from build123d import *

# Parameters (mm, degrees)
SKETCH1_W           = 30
SKETCH1_H           = 11.167486893
SKETCH1_R           = 27.5
SKETCH1_R_2         = 3.25
SKETCH1_R_3         = 12
BOSS_EXTRUDE1_DEPTH = 25.4
SKETCH2_R           = 2.45745
CUT_EXTRUDE1_DEPTH  = 31


with BuildPart() as part:
    # Sketch1 → Boss-Extrude1 (new body)
    # profile 1 of 4: a face of its own
    with BuildSketch(Plane.XY):
        with Locations((-100, -5.583743447)):
            Rectangle(SKETCH1_W, SKETCH1_H)
    # profile 2 of 4: a face of its own
    with BuildSketch(Plane.XY):
        with BuildLine():
            Line((-85, -11.167486893), (-85, -37.625000004))
            ThreePointArc((-85, -37.625000004), (-57.5, -10.125000004), (-30, -37.625000004))
            Line((-30, -37.625000004), (-30, -11.167486893))
            Line((-30, -11.167486893), (-30, 0))
            Line((-30, 0), (-85, 0))
            Line((-85, 0), (-85, -11.167486893))
        make_face()
    # profile 3 of 4: a face of its own
    with BuildSketch(Plane.XY):
        with Locations((-57.5, -37.625000004)):
            Circle(SKETCH1_R)
        with Locations((-58.583096057, -15.151083947)):
            Circle(SKETCH1_R_2, mode=Mode.SUBTRACT)
        with Locations((-38.578565801, -25.450053276)):
            Circle(SKETCH1_R_2, mode=Mode.SUBTRACT)
        with Locations((-37.495469744, -47.923969333)):
            Circle(SKETCH1_R_2, mode=Mode.SUBTRACT)
        with Locations((-56.416903943, -60.098916061)):
            Circle(SKETCH1_R_2, mode=Mode.SUBTRACT)
        with Locations((-76.421434199, -49.799946732)):
            Circle(SKETCH1_R_2, mode=Mode.SUBTRACT)
        with Locations((-77.504530256, -27.326030675)):
            Circle(SKETCH1_R_2, mode=Mode.SUBTRACT)
        with Locations((-57.5, -37.625000004)):
            Circle(SKETCH1_R_3, mode=Mode.SUBTRACT)
    # profile 4 of 4: a face of its own
    with BuildSketch(Plane.XY):
        with Locations((-15, -5.583743447)):
            Rectangle(SKETCH1_W, SKETCH1_H)
    extrude(amount=BOSS_EXTRUDE1_DEPTH)

    # Sketch2 → Cut-Extrude1 (cut)
    with BuildSketch(Plane(origin=(0, 0, 0), x_dir=(1, 0, 0), z_dir=(0, 1, 0))):
        with Locations(Location((-93.73, -12.7, 0), (0, 0, 270))):
            Circle(SKETCH2_R)
        with Locations(Location((-106.43, -12.7, 0), (0, 0, 270))):
            Circle(SKETCH2_R)
        with Locations(Location((-17.53, -12.7, 0), (0, 0, 270))):
            Circle(SKETCH2_R)
        with Locations(Location((-4.83, -12.7, 0), (0, 0, 270))):
            Circle(SKETCH2_R)
    extrude(amount=-CUT_EXTRUDE1_DEPTH, mode=Mode.SUBTRACT)


solid = part.part
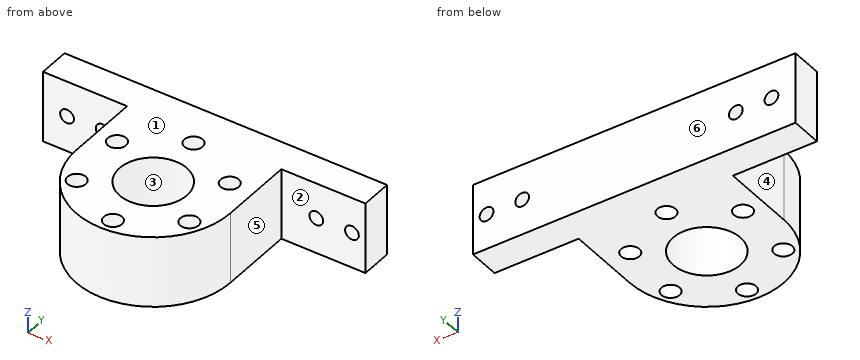
CAD build for the part. Positions are in the model's coordinates, mm. Face numbers are marked on the shaded views. A direction names the side the tool comes from. Round coordinates to 2 decimals unless told otherwise and drop trailing zeros. Write each loop counter-clockwise with the first axis right and the second up, starting at its lowest first coordinate (ties: lowest second). Pieces come first, ordered by that corner, then holes. Notation, with made-up numbers: M 65.5,-27 L 123.5,-27 A23 cw 123.5,-8 Z; hole C 2.5,-2 d9. An arc over 180 degrees is marked long. Use a Markdown table: item, result. Add a question column.
1. Slice it at A-A on x = -106.43. Give the cut face in (y, z).
2. Flat gauge pins, fed straight in: P1, Ø12, axis at x = -35.5, z = 11.5, coming from the -Y side; P2, Ø2, axis at y = -28, z = 13.5, coming from the -X side; P3, Ø12, axis at x = -93, y = -46.5, coming from the -Z side; P4, Ø6.5, axis at x = -17.53, z = 12.7, coming from the -Y side. Where does each tip first touch, or does it go through?
3. Pull direction Y, two halves, no side cores. Call the marked faces 1, 2 and 3: released by +Y, released by -Y, zero draft, split by the parting line, or undercut.
4. Drill centre lines: probe 1 along X at (y, z) = (-4, 12.7); probe 2 along Y at (x, z) = (-57.5, 12.5) (3 decimals); probe 3 along Y at (x, z) = (-55, 21.25). Where is each one in solid material? Low to high.
5. 3-axis set-ups, long thin cutter, end or side, ignore diameter. For the marked faces 4, 5 and 6: which of +Z, -Z, +X, -X, +Y, -Y reach the whole face in a straight line?
6. Slice it at C-C on x = -78. Give the cut face in (y, z), then the cut area to 3 significant figures.
7. Slice it at D-D on y = -35.5. Give the cut face in (x, z), then the cut area to 3 significant figures.
8. Slice it at B-B on y = -4.5. Give the cut face in (x, z), then the cut area to 3 significant figures.
Reply:
| question | item | result |
|---|---|---|
| 1 | outline | M -11.17,0 L 0,0 L 0,10.24 L -11.17,10.24 Z; M -11.17,15.16 L 0,15.16 L 0,25.4 L -11.17,25.4 Z |
| 2 | P1 | stops at y = -59.99 |
| 2 | P2 | stops at x = -85 |
| 2 | P3 | passes through |
| 2 | P4 | stops at y = -11.17 |
| 3 | face 1 | zero draft |
| 3 | face 2 | released by -Y |
| 3 | face 3 | undercut |
| 4 | probe 1 | x = -115 to -108.89, -103.97 to -96.19, -91.27 to -19.99, -15.07 to -7.29, -2.37 to 0 |
| 4 | probe 2 | y = -65.125 to -63.163, -57.035 to -49.625, -25.625 to -18.215, -12.087 to 0 |
| 4 | probe 3 | y = -65.01 to -63.02, -57.17 to -49.36, -25.89 to 0 |
| 5 | face 4 | +Z, -Z, -X, -Y |
| 5 | face 5 | +Z, -Z, +X, -Y |
| 5 | face 6 | +Z, -Z, +X, -X, +Y |
| 6 | outline | M -55.96,0 L -52.64,0 L -52.64,25.4 L -55.96,25.4 Z; M -46.96,0 L -30.54,0 L -30.54,25.4 L -46.96,25.4 Z; M -24.11,0 L 0,0 L 0,25.4 L -24.11,25.4 Z |
| 6 | area | 1,110 mm^2 |
| 7 | outline | M -85,0 L -69.31,0 L -69.31,25.4 L -85,25.4 Z; M -45.69,0 L -30,0 L -30,25.4 L -45.69,25.4 Z |
| 7 | area | 797 mm^2 |
| 8 | outline | M -115,0 L 0,0 L 0,25.4 L -115,25.4 Z; hole C -106.43,12.7 d4.91; hole C -93.73,12.7 d4.91; hole C -17.53,12.7 d4.91; hole C -4.83,12.7 d4.91 |
| 8 | area | 2,850 mm^2 |
